Can you work these out from the model? Positions are in its coordinate system, mm. Face numbers are marked on the shaded views. A direction names the side the tool comes from. Coordinates: 2 decimals unless noted, no trailing zeros. Order: outer loops, then holes, each group sorted by start corner. A loop starts at its lowest first (then second) coordinate and runs counter-clockwise, first axis right, second up. Notation, with made-up numbers: (-15, -32) -> (43, -32) arc R24 cw to (43, -17) -> close; hole circle Ø1 at (32.5, -12). An arc over 180 degrees is marked (long way). Answer in a Markdown table with one row per item. Add a question column.
1. If I drill on line 1 along Z through (x, y) = (-21, -21) (3 decimals); line 2 along X through (y, z) = (1.5, -11.5) (3 decimals), over which ranges is the centre line in solid material (lowest first)? Write a range as [from, to].
2. Imagine slicing it at C-C on y = -10.5. Write out the boundary of the cut face in (x, z) (3 decimals).
3. Will these pins go through, and if not, where does the flat tip stop? pin 1 (3 mm diameter, centred on x = 34.5, z = -36.5, fed in from -Y); pin 2 (4 mm diameter, centred on x = -34.925, z = -34.925, fed in from +Y); pin 3 (2.5 mm diameter, centred on y = -17.5, z = -27.5, fed in from +X); pin 4 (1.5 mm diameter, centred on y = -14.5, z = -15, fed in from -X).
4. We'd pull the mould along Z, two halves only. Please class the marked faces 1, 2 and 3: pulls with the +Z half, pulls with the -Z half, needs draft (parallel to the pull), parting line crosses it, or undercut.
5. Imagine slicing it at D-D on z = -30. Write out the boundary of the cut face in (x, y) (1 decimal).
6. On a 3-axis mill with a long thin cutter (end or side, diameter ignored), from which of +Z, -Z, +X, -X, +Y, -Y can I reach the whole of each face in a straight line? I mean the marked faces 4, 5, 6, 7 and 8. Say none if no direction works.
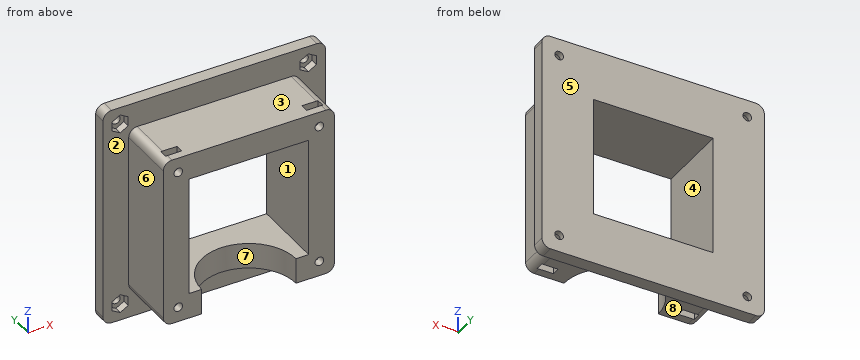
from build123d import *

# Parameters (mm, degrees)
SKETCH1_W               = 82.55
SKETCH1_H               = 82.55
SKETCH1_R               = 1.6
SKETCH1_W_2             = 44.45
SKETCH1_H_2             = 44.45
BOSS_EXTRUDE1_DEPTH     = 4.7625
SKETCH2_W               = 63.5
SKETCH2_H               = 63.5
SKETCH2_W_2             = 44.45
SKETCH2_H_2             = 44.45
BOSS_EXTRUDE2_DEPTH     = 6.35
SKETCH3_W               = 63.5
SKETCH3_H               = 63.5
SKETCH3_W_2             = 44.45
SKETCH3_H_2             = 44.45
BOSS_EXTRUDE3_DEPTH     = 15.875
CUT_EXTRUDE1_REACH      = 75.025
SKETCH4_R               = 17.5
FILLET1_R               = 3.175
CUT_EXTRUDE3_START      = -3
CUT_EXTRUDE3_DEPTH      = 3
SKETCH6_R               = 1.6
CUT_EXTRUDE4_DEPTH      = 7
MIRROR2_START           = -3
MIRROR2_COPY_1_DEPTH    = 3
MIRROR2_COPY_2_SKETCH_R = 1.6
MIRROR2_COPY_2_DEPTH    = 7
CUT_EXTRUDE5_DEPTH      = 2.7625


with BuildPart() as part:
    # Sketch1 → Boss-Extrude1 (new body)
    with BuildSketch(Plane(origin=(0, 0, 0), x_dir=(1, 0, 0), z_dir=(0, 1, 0))):
        Rectangle(SKETCH1_W, SKETCH1_H)
        with Locations((-34.925, 34.925)):
            Circle(SKETCH1_R, mode=Mode.SUBTRACT)
        with Locations((34.925, 34.925)):
            Circle(SKETCH1_R, mode=Mode.SUBTRACT)
        with Locations((34.925, -34.925)):
            Circle(SKETCH1_R, mode=Mode.SUBTRACT)
        with Locations((-34.925, -34.925)):
            Circle(SKETCH1_R, mode=Mode.SUBTRACT)
        Rectangle(SKETCH1_W_2, SKETCH1_H_2, mode=Mode.SUBTRACT)
    extrude(amount=BOSS_EXTRUDE1_DEPTH)

    # Sketch2 → Boss-Extrude2 (add)
    with BuildSketch(Plane.XZ):
        Rectangle(SKETCH2_W, SKETCH2_H)
        Rectangle(SKETCH2_W_2, SKETCH2_H_2, mode=Mode.SUBTRACT)
    extrude(amount=BOSS_EXTRUDE2_DEPTH)

    # Sketch3 → Boss-Extrude3 (add)
    with BuildSketch(Plane.XZ.offset(6.35)):
        Rectangle(SKETCH3_W, SKETCH3_H)
        Rectangle(SKETCH3_W_2, SKETCH3_H_2, mode=Mode.SUBTRACT)
    extrude(amount=BOSS_EXTRUDE3_DEPTH)

    # Sketch4 → Cut-Extrude1 (cut, up to next)
    with BuildSketch(Plane(origin=(0, 0, -31.75), x_dir=(-1, 0, 0), z_dir=(0, 0, -1)), mode=Mode.PRIVATE) as cut_extrude1_sk1:
        with Locations((0, -22.225)):
            Circle(SKETCH4_R)
    cut_extrude1_tool1 = extrude(cut_extrude1_sk1.sketch, amount=-CUT_EXTRUDE1_REACH, mode=Mode.PRIVATE) & part.part
    add(cut_extrude1_tool1.solids().sort_by_distance((0, -22.225, -31.75))[0], mode=Mode.SUBTRACT)

    # Fillet1
    fillet1_edges = [part.edges().sort_by_distance(p)[0] for p in [
        (31.75, -11.1125, -31.75),
        (31.75, -11.1125, 31.75),
        (-31.75, -11.1125, 31.75),
        (-31.75, -11.1125, -31.75),
        (41.275, 2.38125, 41.275),
        (-41.275, 2.38125, 41.275),
        (-41.275, 2.38125, -41.275),
        (41.275, 2.38125, -41.275),
    ]]
    fillet(fillet1_edges, radius=FILLET1_R)

    # Sketch5 → Cut-Extrude3 (cut)
    with BuildSketch(Plane.XZ.offset(22.225).offset(CUT_EXTRUDE3_START)):
        Polygon((-23.19375, -27.925800808), (-23.19375, -24.461699192), (-26.19375, -22.729648385), (-29.19375, -24.461699192), (-29.19375, -27.925800808), (-29.19375, -31.75), (-23.19375, -31.75), align=None)
    cut_extrude3 = extrude(amount=-CUT_EXTRUDE3_DEPTH, mode=Mode.SUBTRACT)

    # Sketch6 → Cut-Extrude4 (cut, through all)
    with BuildSketch(Plane(origin=(0, -16.225, 0), x_dir=(-1, 0, 0), z_dir=(0, -1, 0))):
        with Locations((26.19375, 26.19375)):
            Circle(SKETCH6_R)
    cut_extrude4 = extrude(amount=CUT_EXTRUDE4_DEPTH, mode=Mode.SUBTRACT)

    # Mirror1: Cut-Extrude3, Cut-Extrude4 across plane
    add(cut_extrude3.mirror(Plane(origin=(0, 0, 0), x_dir=(0, 0, 1), z_dir=(1, 0, 0))), mode=Mode.SUBTRACT)
    add(cut_extrude4.mirror(Plane(origin=(0, 0, 0), x_dir=(0, 0, 1), z_dir=(1, 0, 0))), mode=Mode.SUBTRACT)

    # Mirror2: Cut-Extrude4, Cut-Extrude3 across plane
    add(cut_extrude4.mirror(Plane.XY), mode=Mode.SUBTRACT)
    add(cut_extrude3.mirror(Plane.XY), mode=Mode.SUBTRACT)

    # Mirror2 copy 1 sketch → Mirror2 copy 1 (cut)
    with BuildSketch(Plane(origin=(0, -22.225, 0), x_dir=(-1, 0, 0), z_dir=(0, -1, 0)).offset(MIRROR2_START)):
        Polygon((-23.19375, -27.925800808), (-23.19375, -24.461699192), (-26.19375, -22.729648385), (-29.19375, -24.461699192), (-29.19375, -27.925800808), (-29.19375, -31.75), (-23.19375, -31.75), align=None)
    extrude(amount=-MIRROR2_COPY_1_DEPTH, mode=Mode.SUBTRACT)

    # Mirror2 copy 2 sketch → Mirror2 copy 2 (cut, through all)
    with BuildSketch(Plane.XZ.offset(16.225)):
        with Locations((26.19375, 26.19375)):
            Circle(MIRROR2_COPY_2_SKETCH_R)
    extrude(amount=MIRROR2_COPY_2_DEPTH, mode=Mode.SUBTRACT)

    # Sketch7 → Cut-Extrude5 (cut)
    with BuildSketch(Plane(origin=(0, 0, 0), x_dir=(-1, 0, 0), z_dir=(0, -1, 0))):
        Polygon((34.925, -31.460898385), (31.925, -33.192949192), (31.925, -36.657050808), (34.925, -38.389101615), (37.925, -36.657050808), (37.925, -33.192949192), align=None)
        Polygon((-37.925, -33.192949192), (-37.925, -36.657050808), (-34.925, -38.389101615), (-31.925, -36.657050808), (-31.925, -33.192949192), (-34.925, -31.460898385), align=None)
        Polygon((-37.925, 36.657050808), (-37.925, 33.192949192), (-34.925, 31.460898385), (-31.925, 33.192949192), (-31.925, 36.657050808), (-34.925, 38.389101615), align=None)
        Polygon((31.925, 36.657050808), (31.925, 33.192949192), (34.925, 31.460898385), (37.925, 33.192949192), (37.925, 36.657050808), (34.925, 38.389101615), align=None)
    extrude(amount=-CUT_EXTRUDE5_DEPTH, mode=Mode.SUBTRACT)


solid = part.part
Answers follow:
| question | item | result |
|---|---|---|
| 1 | line 1 | z = [-31.75, -22.225], [22.225, 31.75] |
| 1 | line 2 | x = [-41.275, -22.225], [22.225, 41.275] |
| 2 | outline | (-31.75, -28.575) arc R3.175 ccw to (-28.575, -31.75) -> (-12.991, -31.75) -> (-12.991, -22.225) -> (-22.225, -22.225) -> (-22.225, 22.225) -> (22.225, 22.225) -> (22.225, -22.225) -> (12.991, -22.225) -> (12.991, -31.75) -> (28.575, -31.75) arc R3.175 ccw to (31.75, -28.575) -> (31.75, 28.575) arc R3.175 ccw to (28.575, 31.75) -> (-28.575, 31.75) arc R3.175 ccw to (-31.75, 28.575) -> close |
| 3 | pin 1 | stops at y = 0 |
| 3 | pin 2 | stops at y = 4.76 |
| 3 | pin 3 | stops at x = 31.75 |
| 3 | pin 4 | stops at x = -31.75 |
| 4 | face 1 | undercut |
| 4 | face 2 | needs draft |
| 4 | face 3 | pulls with the +Z half |
| 5 | outline | (-41.3, 0) -> (-31.4, 0) -> (-31.4, -22.2) -> (-17.5, -22.2) arc R17.5 cw to (17.5, -22.2) -> (31.4, -22.2) -> (31.4, 0) -> (41.3, 0) -> (41.3, 4.8) -> (-41.3, 4.8) -> close; hole (-29.2, -19.2) -> (-23.2, -19.2) -> (-23.2, -16.2) -> (-29.2, -16.2) -> close; hole (23.2, -19.2) -> (29.2, -19.2) -> (29.2, -16.2) -> (23.2, -16.2) -> close |
| 6 | face 4 | +Y, -Y |
| 6 | face 5 | +Z, -Z, +X, -X, +Y |
| 6 | face 6 | +Z, -Z, -X, -Y |
| 6 | face 7 | -Z, -Y |
| 6 | face 8 | -Z, +X, -X, -Y |
